Geometry check sheet. Reference: drawing and pictorial views, mm from the part's lowest x, y, z. A direction names the side the tool comes from. Round coordinates to 2 decimals unless told otherwise and drop trailing zeros. Loops run counter-clockwise (first coordinate to the right, second up) from the corner with the lowest first, then second, coordinate; pieces in that order, holes last. Notation, with made-up numbers: M -1.5,74.5 L 16.5,74.5 A10 ccw 16.5,78.5 Z; hole C 5.25,11.5 d2. An arc over 180 degrees is marked long. One line per question, with ' | ' between items. Start each with the question number.
(1) Section check D-D (y = 30.6). Record the boundary of the cut face in (x, z), and give its area (3 significant figures).
(2) Section check B-B (z = 1.75). Record the boundary of the cut face in (x, y), and give its area (3 significant figures).
(3) Section check A-A (y = 2.5). Record the boundary of the cut face in (x, z).
(4) Draft check along X on the marked faces 1, 2, 3 and 4. Enter one of: +X half, -X half, draft (parallel to the pull), parting line (faces both ways), or undercut.
(5) Tool access check on the marked faces 5 and 6. Record the directions out of +Z, -Z, +X, -X, +Y, -Y that give a thin tool (end or side, any length) a straight path to the whole face; none if there is none.
(6) Section check C-C (x = 9). Record the boundary of the cut face in (y, z), and give its area (3 significant figures).
(7) Go/stop test with flat-tipped pins: P1, Ø1, axis at y = 4, z = 2, coming from the -X side; P2, Ø3.5, axis at y = 13, z = 4, coming from the +X side. Record where each tip stops, or that it passes through.
(8) Thickness scan on probe 1 along X at (y, z) = (2.5, 1.75); probe 2 along Y at (x, z) = (10.5, 5); probe 3 along X at (y, z) = (2.5, 2.5). Record the ranges inside material, lowest first. Write a range as [from, to].
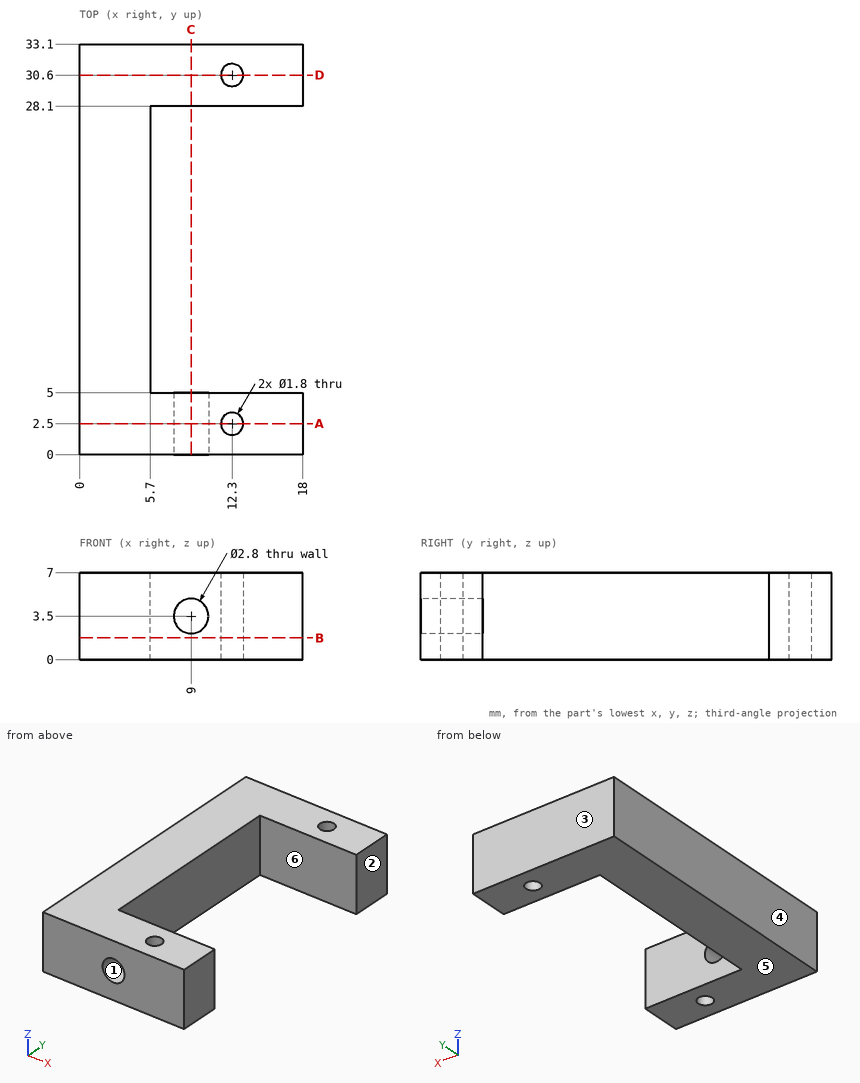
The answers:
1) outline: M 0,0 L 11.4,0 L 11.4,7 L 0,7 Z; M 13.2,0 L 18,0 L 18,7 L 13.2,7 Z | area: 113 mm²
2) outline: M 0,0 L 18,0 L 18,5 L 5.7,5 L 5.7,28.1 L 18,28.1 L 18,33.1 L 0,33.1 Z; hole C 12.3,2.5 d1.8; hole C 12.3,30.6 d1.8 | area: 307 mm²
3) outline: M 0,0 L 11.4,0 L 11.4,7 L 0,7 Z; M 13.2,0 L 18,0 L 18,7 L 13.2,7 Z; hole C 9,3.5 d2.8
4) face 1: undercut | face 2: +X half | face 3: draft | face 4: -X half
5) face 5: -Z, +X, -X, +Y, -Y | face 6: +Z, -Z, +X
6) outline: M 0,0 L 5,0 L 5,2.1 L 0,2.1 Z; M 0,4.9 L 5,4.9 L 5,7 L 0,7 Z; M 28.1,0 L 33.1,0 L 33.1,7 L 28.1,7 Z | area: 56.0 mm²
7) P1: x = 0 | P2: x = 5.7
8) probe 1: [0, 11.4], [13.2, 18] | probe 2: [0, 5], [28.1, 33.1] | probe 3: [0, 8.02], [9.98, 11.4], [13.2, 18]
